```python
from build123d import *

# Parameters (mm, degrees)
BOSS_EXTRUDE1_DEPTH      = 50
BOSS_EXTRUDE1_DEPTH_BACK = 50
SKETCH1_W                = 200
SKETCH1_H                = 152.061
SHELL1_T                 = -5
SKETCH3_W                = 190
SKETCH3_H                = 142.061
BOSS_EXTRUDE2_DEPTH      = 37
CUT_EXTRUDE1_REACH       = 221.729
SKETCH2_W                = 36
SKETCH2_H                = 58
SKETCH4_W                = 36
SKETCH4_H                = 46.5
SKETCH4_R                = 2
CUT_EXTRUDE2_DEPTH       = 2
SKETCH4_3_R              = 2
CUT_EXTRUDE3_DEPTH       = 139.364146115
SKETCH5_W                = 169.952904784
SKETCH5_H                = 5
CUT_EXTRUDE4_DEPTH       = 63
CUT_EXTRUDE5_START       = -37
CUT_EXTRUDE5_DEPTH       = 37
SKETCH9_R                = 1.2
SKETCH9_R_2              = 1.5
CUT_EXTRUDE6_DEPTH       = 10
CUT_EXTRUDE7_DEPTH       = 102
FILLET1_R                = 10
SKETCH11_W               = 62
SKETCH11_H               = 5
BOSS_EXTRUDE3_DEPTH      = 100
SKETCH12_W               = 57
SKETCH12_H               = 3
SKETCH12_W_2             = 43
SKETCH12_H_2             = 2
CUT_EXTRUDE8_DEPTH       = 91
SKETCH13_W               = 57
SKETCH13_H               = 3
CUT_EXTRUDE9_DEPTH       = 7
FILLET2_R                = 10
FILLET3_R                = 100
SKETCH15_R               = 5
CUT_EXTRUDE10_DEPTH      = 28
SKETCH17_R               = 4.2
SKETCH17_R_2             = 4.5
CUT_EXTRUDE11_DEPTH      = 2.5


# Read off the part's stored shape, not the designer's step: Cut-Extrude5
with BuildPart() as part:
    # Sketch1 → Boss-Extrude1 (new, two sides: drawn at the far end of the back side and taken through both)
    with BuildSketch(Plane(origin=(0, 0, 0), x_dir=(1, 0, 0), z_dir=(0, 1, 0)).offset(-BOSS_EXTRUDE1_DEPTH_BACK)):
        Rectangle(SKETCH1_W, SKETCH1_H)
    extrude(amount=BOSS_EXTRUDE1_DEPTH + BOSS_EXTRUDE1_DEPTH_BACK)

    # Shell1
    shell1_openings = [part.faces().sort_by_distance(p)[0] for p in [
        (0, -50, 0),
    ]]
    offset(amount=SHELL1_T, openings=shell1_openings, kind=Kind.INTERSECTION)

    # Sketch3 → Boss-Extrude2 (add)
    with BuildSketch(Plane.XZ.offset(-45)):
        Rectangle(SKETCH3_W, SKETCH3_H)
    extrude(amount=BOSS_EXTRUDE2_DEPTH)

    # Sketch2 → Cut-Extrude1 (cut, up to next)
    with BuildSketch(Plane.ZY.offset(100), mode=Mode.PRIVATE) as cut_extrude1_sk1:
        with Locations((-46.0305, -21)):
            Rectangle(SKETCH2_W, SKETCH2_H)
    cut_extrude1_tool1 = extrude(cut_extrude1_sk1.sketch, amount=-CUT_EXTRUDE1_REACH, mode=Mode.PRIVATE) & part.part
    cut_extrude1 = cut_extrude1_tool1.solids().sort_by_distance((-100, -21, -46.0305))[0]
    add(cut_extrude1, mode=Mode.SUBTRACT)

    # Mirror1: Cut-Extrude1 across plane
    add(cut_extrude1.mirror(Plane(origin=(0, 0, 0), x_dir=(0, 0, 1), z_dir=(1, 0, 0))), mode=Mode.SUBTRACT)

    # Sketch4 → Cut-Extrude2 (cut)
    with BuildSketch(Plane.XZ.offset(-8)):
        with Locations((-59, -34.0305)):
            Rectangle(SKETCH4_W, SKETCH4_H)
        with Locations(Location((-48, -50.2805, 0), (0, 0, 270))):
            Circle(SKETCH4_R, mode=Mode.SUBTRACT)
        with Locations(Location((-70, -50.2805, 0), (0, 0, 270))):
            Circle(SKETCH4_R, mode=Mode.SUBTRACT)
        with Locations(Location((-48, -17.7805, 0), (0, 0, 270))):
            Circle(SKETCH4_R, mode=Mode.SUBTRACT)
        with Locations(Location((-70, -17.7805, 0), (0, 0, 270))):
            Circle(SKETCH4_R, mode=Mode.SUBTRACT)
    cut_extrude2 = extrude(amount=-CUT_EXTRUDE2_DEPTH, mode=Mode.SUBTRACT)

    # Sketch4<3> → Cut-Extrude3 (cut, through all)
    with BuildSketch(Plane.XZ.offset(-8)):
        with BuildLine():
            Line((-70, -19.7805), (-70, -17.7805))
            Line((-70, -17.7805), (-68, -17.7805))
            ThreePointArc((-68, -17.7805), (-71.414213562, -16.366286438), (-70, -19.7805))
        make_face()
        with BuildLine():
            Line((-68, -17.7805), (-70, -17.7805))
            Line((-70, -17.7805), (-70, -19.7805))
            ThreePointArc((-70, -19.7805), (-68.585786438, -19.194713562), (-68, -17.7805))
        make_face()
        with Locations(Location((-48, -17.7805, 0), (0, 0, 270))):
            Circle(SKETCH4_3_R)
        with Locations(Location((-70, -50.2805, 0), (0, 0, 270))):
            Circle(SKETCH4_3_R)
        with Locations(Location((-48, -50.2805, 0), (0, 0, 270))):
            Circle(SKETCH4_3_R)
    cut_extrude3 = extrude(amount=-CUT_EXTRUDE3_DEPTH, mode=Mode.SUBTRACT)

    # Mirror2: Cut-Extrude2, Cut-Extrude3 across plane
    add(cut_extrude2.mirror(Plane(origin=(0, 0, 0), x_dir=(0, 0, 1), z_dir=(1, 0, 0))), mode=Mode.SUBTRACT)
    add(cut_extrude3.mirror(Plane(origin=(0, 0, 0), x_dir=(0, 0, 1), z_dir=(1, 0, 0))), mode=Mode.SUBTRACT)

    # Sketch5 → Cut-Extrude4 (cut)
    with BuildSketch(Plane.XZ.offset(-8)):
        with Locations((10.023547608, 73.5305)):
            Rectangle(SKETCH5_W, SKETCH5_H)
    extrude(amount=CUT_EXTRUDE4_DEPTH, mode=Mode.SUBTRACT)

    # Cut-Extrude5 outline → Cut-Extrude5 (cut)
    with BuildSketch(Plane.XZ.offset(-8).offset(CUT_EXTRUDE5_START)):
        Polygon((-41, -10.7805), (-41, -71.0305), (41, -71.0305), (41, -10.7805), (71.419165144, -10.7805), (71.419165144, 76.0305), (-74.952904784, 76.0305), (-74.952904784, 71.0305), (-77, 71.0305), (-77, -10.7805), align=None)
    extrude(amount=CUT_EXTRUDE5_DEPTH, mode=Mode.SUBTRACT)

    # Sketch9 → Cut-Extrude6 (cut)
    with BuildSketch(Plane.XZ.offset(-45)):
        with Locations(Location((37.2, -68.0305, 0), (0, 0, 270))):
            Circle(SKETCH9_R)
        with Locations(Location((-37.2, -68.0305, 0), (0, 0, 270))):
            Circle(SKETCH9_R)
        with Locations(Location((37.2, -2.0305, 0), (0, 0, 270))):
            Circle(SKETCH9_R)
        with Locations(Location((-37.2, -2.0305, 0), (0, 0, 270))):
            Circle(SKETCH9_R)
        with Locations(Location((0, -35.0305, 0), (0, 0, 270))):
            Circle(SKETCH9_R_2)
    extrude(amount=-CUT_EXTRUDE6_DEPTH, mode=Mode.SUBTRACT)

    # Sketch10 → Cut-Extrude7 (cut)
    with BuildSketch(Plane.XZ.offset(50)):
        Polygon((0, 76.0305), (100, 49.235580757), (100, 76.0305), align=None)
    cut_extrude7 = extrude(amount=-CUT_EXTRUDE7_DEPTH, mode=Mode.SUBTRACT)

    # Mirror3: Cut-Extrude7 across plane
    add(cut_extrude7.mirror(Plane(origin=(0, 0, 0), x_dir=(0, 0, 1), z_dir=(1, 0, 0))), mode=Mode.SUBTRACT)

    # Fillet1
    fillet1_edges = [part.edges().sort_by_distance(p)[0] for p in [
        (0, 47.5, 76.0305),
    ]]
    fillet(fillet1_edges, radius=FILLET1_R)

    # Sketch11 → Boss-Extrude3 (add)
    with BuildSketch(Plane.XZ.offset(50)):
        Polygon((85, -86.0305), (85, -76.0305), (-85, -76.0305), (-85, -86.0305), (-31, -86.0305), (31, -86.0305), align=None)
        with Locations((0, -88.5305)):
            Rectangle(SKETCH11_W, SKETCH11_H)
    extrude(amount=-BOSS_EXTRUDE3_DEPTH)

    # Sketch12 → Cut-Extrude8 (cut)
    with BuildSketch(Plane.XZ.offset(50)):
        with Locations((0, -87.5305)):
            Rectangle(SKETCH12_W, SKETCH12_H)
        with Locations((0, -90.0305)):
            Rectangle(SKETCH12_W_2, SKETCH12_H_2)
    extrude(amount=-CUT_EXTRUDE8_DEPTH, mode=Mode.SUBTRACT)

    # Sketch13 → Cut-Extrude9 (cut)
    with BuildSketch(Plane.XZ.offset(-41)):
        with Locations((0, -87.5305)):
            Rectangle(SKETCH13_W, SKETCH13_H)
    extrude(amount=-CUT_EXTRUDE9_DEPTH, mode=Mode.SUBTRACT)

    # Fillet2
    fillet2_edges = [part.edges().sort_by_distance(p)[0] for p in [
        (-100, 0, -76.0305),
        (100, 0, -76.0305),
    ]]
    fillet(fillet2_edges, radius=FILLET2_R)

    # Fillet3
    # the kernel refuses this fillet: 100 mm, written as the material it takes off along each edge
    with BuildSketch(Plane(origin=(-85, -158.972473589, -86.0305), x_dir=(0, 0, 1), z_dir=(0, 1, 0))) as fillet3_piece_1:
        with BuildLine():
            CenterArc((100, 43.588989435), FILLET3_R, 180, 25.841932763)
            Line((0, 43.588989435), (-2, 43.588989435))
            Line((-2, 43.588989435), (-2, 0))
            Line((-2, 0), (0, -2))
            ThreePointArc((0, -2), (5, -2), (8.2, -0.871779789))
            Line((8.2, -0.871779789), (10, 0))
        make_face()
    extrude(amount=317.944947177, mode=Mode.SUBTRACT)
    with BuildSketch(Plane(origin=(85, -158.972473589, -86.0305), x_dir=(0, 0, 1), z_dir=(0, 1, 0))) as fillet3_piece_2:
        with BuildLine():
            CenterArc((100, -43.588989435), FILLET3_R, 154.158067237, 25.841932763)
            Line((0, -43.588989435), (-2, -43.588989435))
            Line((-2, -43.588989435), (-2, 0))
            Line((-2, 0), (0, 2))
            ThreePointArc((0, 2), (5, 2), (8.2, 0.871779789))
            Line((8.2, 0.871779789), (10, 0))
        make_face()
    extrude(amount=317.944947177, mode=Mode.SUBTRACT)

    # Sketch15 → Cut-Extrude10 (cut)
    with BuildSketch(Plane(origin=(0, 50, 0), x_dir=(1, 0, 0), z_dir=(0, 1, 0))):
        with Locations(Location((70, 17.7805, 0), (0, 0, 270))):
            Circle(SKETCH15_R)
        with Locations(Location((48, 17.7805, 0), (0, 0, 270))):
            Circle(SKETCH15_R)
        with Locations(Location((70, 50.2805, 0), (0, 0, 270))):
            Circle(SKETCH15_R)
        with Locations(Location((-48, 50.2805, 0), (0, 0, 90))):
            Circle(SKETCH15_R)
        with Locations(Location((48, 50.2805, 0), (0, 0, 270))):
            Circle(SKETCH15_R)
        with Locations(Location((-70, 50.2805, 0), (0, 0, 90))):
            Circle(SKETCH15_R)
        with Locations(Location((-48, 17.7805, 0), (0, 0, 90))):
            Circle(SKETCH15_R)
        with Locations(Location((-70, 17.7805, 0), (0, 0, 90))):
            Circle(SKETCH15_R)
    extrude(amount=-CUT_EXTRUDE10_DEPTH, mode=Mode.SUBTRACT)

    # Sketch17 → Cut-Extrude11 (cut)
    with BuildSketch(Plane(origin=(0, 50, 0), x_dir=(1, 0, 0), z_dir=(0, 1, 0))):
        with Locations(Location((-37.2, 2.0305, 0), (0, 0, 270))):
            Circle(SKETCH17_R)
        with Locations(Location((37.2, 68.0305, 0), (0, 0, 270))):
            Circle(SKETCH17_R)
        with Locations(Location((37.2, 2.0305, 0), (0, 0, 270))):
            Circle(SKETCH17_R)
        with Locations(Location((-37.2, 68.0305, 0), (0, 0, 270))):
            Circle(SKETCH17_R)
        with Locations(Location((0, 35.0305, 0), (0, 0, 270))):
            Circle(SKETCH17_R_2)
    extrude(amount=-CUT_EXTRUDE11_DEPTH, mode=Mode.SUBTRACT)


solid = part.part
```
CAD build for the part. Positions are in the model's coordinates, mm. A direction names the side the tool comes from. Give positions to 0.01 mm unless a question says otherwise; leave off trailing zeros. Order: outer loops, then holes, each group sorted by start corner. A loop starts at its lowest first (then second) coordinate and runs counter-clockwise, first axis right, second up.
(1) Saw through at A-A, the plane y = -23.5. State how many separate pieces and enclosed holes the cut face has, then the cut area to 3 significant figures.
(2) Tool access for faces 1 (the flat face through (-23, 13, -89.03)), 2 (the cylindrical face through (-40.926, 48.768, -0.092)), 3 (the flat face through (-95, -21, -67)): list every direction of +Z, -Z, +X, -X, +Y, -Y with a clear straight run to the whole face (end or side of a thin tool).
(3) Drill centre lines: L1, parallel to X at y = 38, z = 49; L2, parallel to X at y = -41, z = 19.5; L3, parallel to Z at x = -70, y = 37.25. Where is each one in solid material? Low to high.
(4) Mould opens along Z. For faces 4 (the cylindrical face through (-0.037, 47.535, 75.678)), 5 (the cylindrical face through (-70.22, 36.196, -45.285)), 6 (the flat face through (-1, 50, -9)), 7 (the flat face through (23, 11, -91.03)) say: released by +Z, released by -Z, zero draft, split by the parting line, or undercut.
(5) Flat gauge pins, fed straight in: pin 1 (1 mm diameter, centred on y = -8, z = -68.5, fed in from -X); pin 2 (8 mm diameter, centred on x = -3, y = 15, fed in from -Z); pin 3 (11.5 mm diameter, centred on x = 48, z = -50.28, fed in from -Y). Where does each tip first touch, or does it go through?
(6) Saw through at C-C, the plane x = 7.5. Give the cut face in (y, z), then the cut area to 3 significant figures.
Results found:
1. separate pieces: 3
1. enclosed holes: 0
1. area: 3,270 mm2
2. face 1: -Y
2. face 2: +Y
2. face 3: +Z, -Y
3. L1: x = -100 to -77, 71.42 to 100
3. L2: x = -100 to -95, 95 to 100
3. L3: z = -81.86 to -55.28, -45.28 to -22.78, -12.78 to -10.78
4. face 4: released by +Z
4. face 5: undercut
4. face 6: zero draft
4. face 7: released by -Z
5. pin 1: stops at x = -99.8
5. pin 2: stops at z = -86.03
5. pin 3: stops at y = 10
6. outline: (-50, -86.03) - (48, -86.03) - (48, -89.03) - (41, -89.03) - (41, -91.03) - (50, -91.03) - (50, 74.02) - (45, 74.02) - (45, -71.03) - (-50, -71.03) - close
6. area: 2,250 mm2
